Here's how the part is built. I have some questions about the finished solid (model axes, mm). Face numbers are marked on the shaded views. Round coordinates to 2 decimals unless told otherwise and drop trailing zeros. Loops run counter-clockwise (first coordinate to the right, second up) from the corner with the lowest first, then second, coordinate; pieces in that order, holes last. Notation, with made-up numbers: (71.5, 44.25) - (119.5, 44.25) arc R9 cw to (119.5, 58.25) - close; hole circle Ø8 at (-4, 39.5). An arc over 180 degrees is marked (long way). Answer as a JSON object with one key per item and string values. Group by question number.
1) I want a section at C-C, the plane y = 4. Please give me the cut outline in (x, z) (3 decimals), then the cut area to 3 significant figures.
2) If we mould it in two halves opening along X, with no side actions, what happens to the marked faces 1 and 2? For each: pulls with the +X half, pulls with the -X half, needs draft (parallel to the pull), parting line crosses it, or undercut.
3) I want a section at A-A, the plane x = 0. Please give me the cut outline in (y, z) (3 decimals), then the cut area to 3 significant figures.
4) I want a section at B-B, the plane z = 0. Please give me the cut outline in (x, y) (3 decimals), then the cut area to 3 significant figures.
5) If I drill on line 1 along Z through (x, y) = (0, 77.25) (3 decimals); line 2 along Z through (x, y) = (0, 66.95) (3 decimals), over which ranges is the centre line in solid material (lowest first)? Write a range as [from, to].
6) I want a section at D-D, the plane z = -27. Please give me the cut outline in (x, y).
7) Will these pins go through, and if not, where does the flat tip stop? P1, Ø6, axis at y = -21.5, z = 37.5, coming from the +X side; P2, Ø1.5, axis at x = -68.5, y = 60.5, coming from the +Z side; P3, Ø12, axis at y = -33.5, z = 28.5, coming from the +X side.
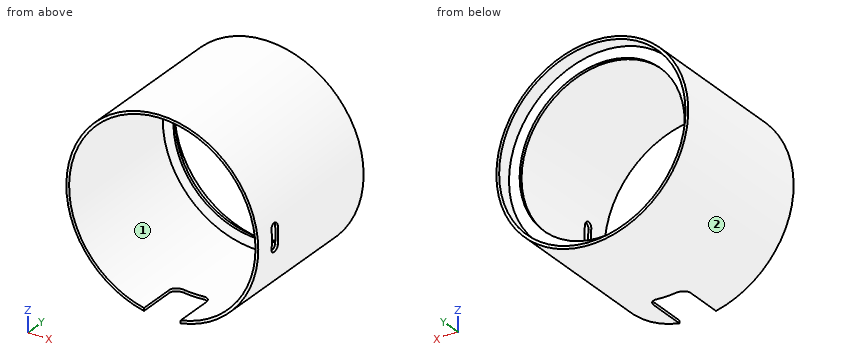
from build123d import *

# Parameters (mm, degrees)
SKETCH1_R           = 104.625
SKETCH1_R_2         = 101.625
BOSS_EXTRUDE1_DEPTH = 83.5
CUT_EXTRUDE1_REACH  = 106.625
SKETCH2_W           = 40
SKETCH2_H           = 50
CUT_EXTRUDE2_REACH  = 106.625
SKETCH4_R           = 101.625
SKETCH4_R_2         = 90
BOSS_EXTRUDE2_DEPTH = 3
FILLET1_R           = 10


with BuildPart() as part:
    # Sketch1 → Boss-Extrude1 (new body, symmetric)
    with BuildSketch(Plane(origin=(0, 0, 0), x_dir=(1, 0, 0), z_dir=(0, 1, 0))):
        Circle(SKETCH1_R)
        Circle(SKETCH1_R_2, mode=Mode.SUBTRACT)
    extrude(amount=BOSS_EXTRUDE1_DEPTH, both=True)

    # Sketch2 → Cut-Extrude1 (cut, up to next)
    with BuildSketch(Plane.XY, mode=Mode.PRIVATE) as cut_extrude1_sk1:
        with Locations((0, -58.5)):
            Rectangle(SKETCH2_W, SKETCH2_H)
    cut_extrude1_tool1 = extrude(cut_extrude1_sk1.sketch, amount=-CUT_EXTRUDE1_REACH, mode=Mode.PRIVATE) & part.part
    add(cut_extrude1_tool1.solids().sort_by_distance((0, -58.5, 0))[0], mode=Mode.SUBTRACT)

    # Sketch3 → Cut-Extrude2 (cut, up to next)
    with BuildSketch(Plane(origin=(0, 0, 0), x_dir=(0, 0, -1), z_dir=(1, 0, 0)), mode=Mode.PRIVATE) as cut_extrude2_sk1:
        with BuildLine():
            Line((-10, -51.809036258), (10, -51.809036258))
            ThreePointArc((10, -51.809036258), (15, -56.809036258), (10, -61.809036258))
            Line((10, -61.809036258), (-10, -61.809036258))
            ThreePointArc((-10, -61.809036258), (-15, -56.809036258), (-10, -51.809036258))
        make_face()
    cut_extrude2_tool1 = extrude(cut_extrude2_sk1.sketch, amount=CUT_EXTRUDE2_REACH, mode=Mode.PRIVATE) & part.part
    add(cut_extrude2_tool1.solids().sort_by_distance((0, -56.809036, 0))[0], mode=Mode.SUBTRACT)

    # Sketch4 → Boss-Extrude2 (add)
    with BuildSketch(Plane(origin=(0, 67.9, 0), x_dir=(1, 0, 0), z_dir=(0, 1, 0))):
        Circle(SKETCH4_R)
        Circle(SKETCH4_R_2, mode=Mode.SUBTRACT)
    extrude(amount=-BOSS_EXTRUDE2_DEPTH)

    # Fillet1
    fillet1_edges = [part.edges().sort_by_distance(p)[0] for p in [
        (20, -33.5, -101.166583758),
        (-20, -33.5, -101.166583758),
    ]]
    fillet(fillet1_edges, radius=FILLET1_R)


solid = part.part
Outcome:
{
 "1": {"outline": "circle Ø209.25 at (0, 0); hole circle Ø203.25 at (0, 0)", "area": "1,940 mm^2"},
 "2": {"face 1": "undercut", "face 2": "parting line crosses it"},
 "3": {"outline": "(-83.5, 101.625) - (64.9, 101.625) - (64.9, 90) - (67.9, 90) - (67.9, 101.625) - (83.5, 101.625) - (83.5, 104.625) - (-83.5, 104.625) - close; (-33.5, -104.625) - (83.5, -104.625) - (83.5, -101.625) - (67.9, -101.625) - (67.9, -90) - (64.9, -90) - (64.9, -101.625) - (-33.5, -101.625) - close", "area": "922 mm^2"},
 "4": {"outline": "(-104.625, -83.5) - (-101.625, -83.5) - (-101.625, 64.9) - (-90, 64.9) - (-90, 67.9) - (-101.625, 67.9) - (-101.625, 83.5) - (-104.625, 83.5) - close; (90, 64.9) - (101.625, 64.9) - (101.625, -51.809) - (104.625, -51.809) - (104.625, 83.5) - (101.625, 83.5) - (101.625, 67.9) - (90, 67.9) - close; (101.625, -83.5) - (104.625, -83.5) - (104.625, -61.809) - (101.625, -61.809) - close", "area": "1,040 mm^2"},
 "5": {"line 1": "[-104.625, -101.625], [101.625, 104.625]", "line 2": "[-104.625, -90], [90, 104.625]"},
 "6": {"outline": "(-101.08, -83.5) - (-97.97, -83.5) - (-97.97, 64.9) - (-85.85, 64.9) - (-85.85, 67.9) - (-97.97, 67.9) - (-97.97, 83.5) - (-101.08, 83.5) - close; (85.85, 64.9) - (97.97, 64.9) - (97.97, -83.5) - (101.08, -83.5) - (101.08, 83.5) - (97.97, 83.5) - (97.97, 67.9) - (85.85, 67.9) - close"},
 "7": {"P1": "x = 98.77", "P2": "z = 79.73", "P3": "x = 102.18"}
}
